Check sheet for the modelled part. Datum: model origin and axes. Units: mm. Round coordinates to 2 decimals unless told otherwise and drop trailing zeros. Loops run counter-clockwise (first coordinate to the right, second up) from the corner with the lowest first, then second, coordinate; pieces in that order, holes last. Notation, with made-up numbers: (6.25, 51) - (35.25, 51) arc R23 cw to (35.25, 69) - close; hole circle Ø7 at (-6, -13). An arc over 180 degrees is marked (long way). Answer in a Markdown table with one row per item. Add a question column.
(1) Cross-section at B-B on x = -4.5. Enter the section's corners in (y, z), then the cut area to 3 significant figures.
(2) Thickness scan on line 1 along X through (y, z) = (20.5, 0.3); line 2 along Y through (x, z) = (-11.5, 1.1); line 3 along Y through (x, z) = (9, 1.5). Record the ranges inside material, lowest first.
(3) Cross-section at A-A on x = 9. Enter the section's corners in (y, z), then the cut area to 3 significant figures.
(4) Cross-section at C-C on z = 0.55. Count the separate pieces of the cut face and the enclosed holes in it, then the cut area to 3 significant figures.
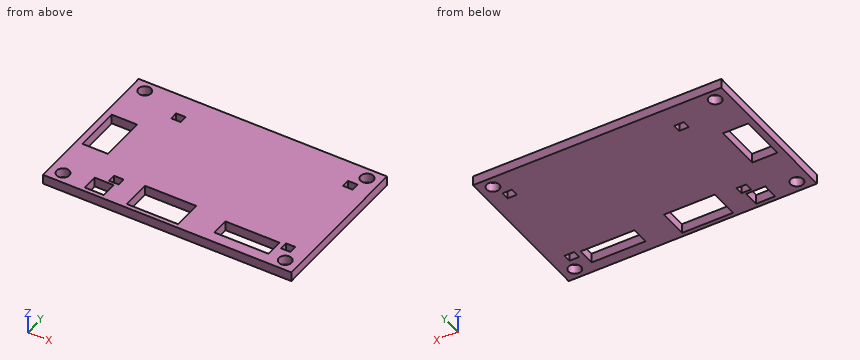
from build123d import *

# Parameters (mm, degrees)
SKETCH1_W           = 41.275
SKETCH1_H           = 25.4
SKETCH1_R           = 1.0541
BOSS_EXTRUDE1_DEPTH = 1.5875
SKETCH2_W           = 9
SKETCH2_H           = 2.93
SKETCH2_W_2         = 8.509
SKETCH2_H_2         = 4.826
SKETCH2_W_3         = 3.175
SKETCH2_H_3         = 2.6162
SKETCH2_W_4         = 4.22
SKETCH2_H_4         = 7.75
SKETCH2_W_5         = 1.5875
SKETCH2_H_5         = 1.3208
CUT_EXTRUDE1_DEPTH  = 1.5875


with BuildPart() as part:
    # Sketch1 → Boss-Extrude1 (new body)
    with BuildSketch(Plane.XY):
        with Locations((0, 12.7)):
            Rectangle(SKETCH1_W, SKETCH1_H)
        with Locations((-18.4658, 23.5585)):
            Circle(SKETCH1_R, mode=Mode.SUBTRACT)
        with Locations((-18.4658, 1.8415)):
            Circle(SKETCH1_R, mode=Mode.SUBTRACT)
        with Locations((18.4658, 1.8415)):
            Circle(SKETCH1_R, mode=Mode.SUBTRACT)
        with Locations((18.4658, 23.5585)):
            Circle(SKETCH1_R, mode=Mode.SUBTRACT)
    extrude(amount=BOSS_EXTRUDE1_DEPTH)

    # Sketch2 → Cut-Extrude1 (cut)
    with BuildSketch(Plane.XY.offset(1.5875)):
        with Locations((11.1858, 3.3045)):
            Rectangle(SKETCH2_W, SKETCH2_H)
        with Locations((-2.8993, 3.1205)):
            Rectangle(SKETCH2_W_2, SKETCH2_H_2)
        with Locations((-12.5513, 2.0156)):
            Rectangle(SKETCH2_W_3, SKETCH2_H_3)
        with Locations((-17.4978, 12.709)):
            Rectangle(SKETCH2_W_4, SKETCH2_H_4)
        with Locations((17.30375, 20.9804)):
            Rectangle(SKETCH2_W_5, SKETCH2_H_5)
        with Locations((17.30375, 4.4704)):
            Rectangle(SKETCH2_W_5, SKETCH2_H_5)
        with Locations((-11.25855, 4.4704)):
            Rectangle(SKETCH2_W_5, SKETCH2_H_5)
        with Locations((-11.25855, 20.9804)):
            Rectangle(SKETCH2_W_5, SKETCH2_H_5)
    extrude(amount=-CUT_EXTRUDE1_DEPTH, mode=Mode.SUBTRACT)


solid = part.part
Answers:
| question | item | result |
|---|---|---|
| 1 | outline | (0, 0) - (0.71, 0) - (0.71, 1.59) - (0, 1.59) - close; (5.53, 0) - (25.4, 0) - (25.4, 1.59) - (5.53, 1.59) - close |
| 1 | area | 32.7 mm^2 |
| 2 | line 1 | x = -20.64 to -12.05, -10.46 to 16.51, 18.1 to 20.64 |
| 2 | line 2 | y = 0 to 0.71, 3.32 to 3.81, 5.13 to 20.32, 21.64 to 25.4 |
| 2 | line 3 | y = 0 to 1.84, 4.77 to 25.4 |
| 3 | outline | (0, 0) - (1.84, 0) - (1.84, 1.59) - (0, 1.59) - close; (4.77, 0) - (25.4, 0) - (25.4, 1.59) - (4.77, 1.59) - close |
| 3 | area | 35.7 mm^2 |
| 4 | separate pieces | 1 |
| 4 | enclosed holes | 12 |
| 4 | area | 918 mm^2 |
